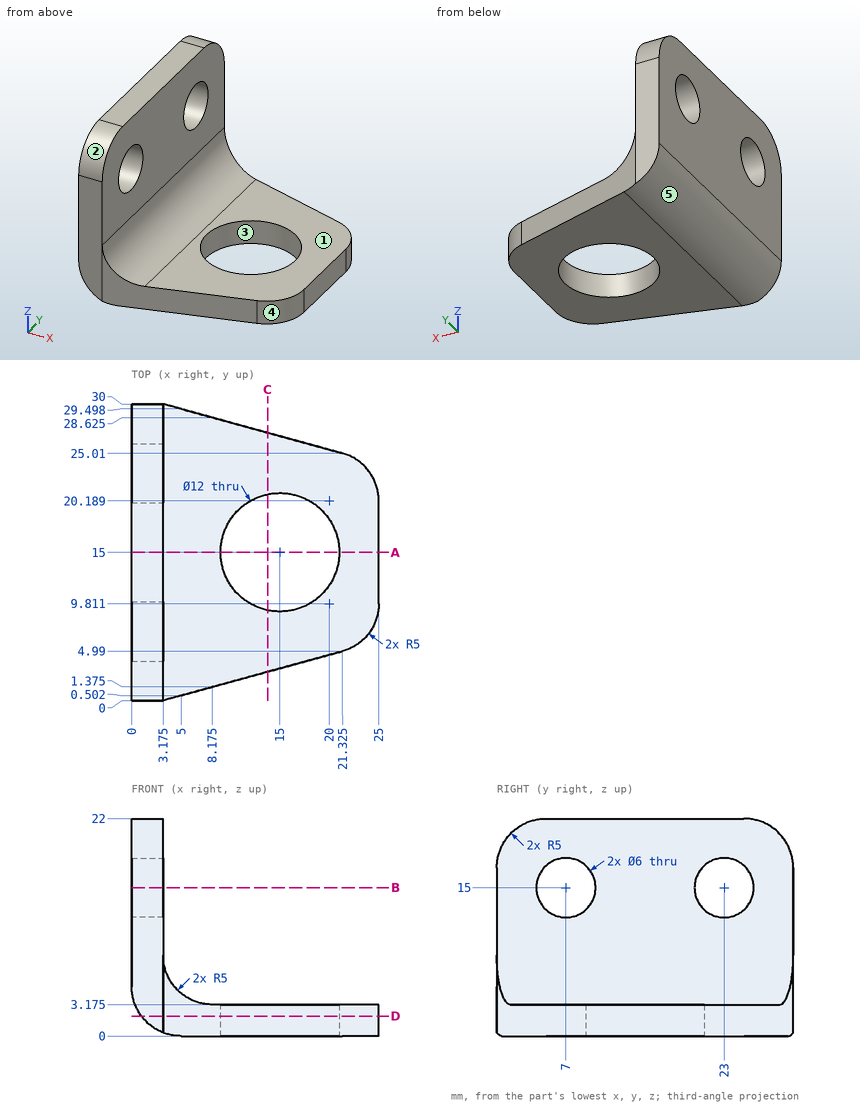
Verification items for this drawing (mm, ordinates from the low corner). A direction names the side the tool comes from. Coordinates: 2 decimals unless noted, no trailing zeros. Loops run counter-clockwise (first coordinate to the right, second up) from the corner with the lowest first, then second, coordinate; pieces in that order, holes last. Notation, with made-up numbers: (76, 10) - (123, 10) arc R5 ccw to (123, 18) - close; hole circle Ø9 at (73.5, 51). An arc over 180 degrees is marked (long way). Use one line per item in the form item = value. Start each with the question number.
Item 1: Gauge pin test, flat ends, axial feed: pin 1 (8 mm diameter, centred on x = 14.5, y = 18.5, fed in from +Z) (3 decimals); pin 2 (8 mm diameter, centred on y = 7, z = 15, fed in from +X) (3 decimals); pin 3 (12 mm diameter, centred on x = 15, z = 15.5, fed in from -Y); pin 4 (5 mm diameter, centred on y = 8, z = 6.5, fed in from +X) (1 decimal). Record the tip position at first contact, or that the pin passes through.
Item 2: Mould release check, pull along X, two halves, no side actions. Record for the marked faces 3, 4 and 5: +X half, -X half, draft (parallel to the pull), parting line (faces both ways), or undercut.
Item 3: Thickness scan on probe 1 along Y at (x, z) = (2.1, 15); probe 2 along X at (y, z) = (8, 19.5) (1 decimal). Record the ranges inside material, lowest first.
Item 4: Section check B-B, the plane z = 15. Enter the section's corners in (x, y) (1 decimal).
Item 5: Section check D-D, the plane z = 2. Enter the section's corners in (x, y) (1 decimal).
Item 6: Tool access check on the marked faces 1 and 2. Record the directions out of +Z, -Z, +X, -X, +Y, -Y that give a thin tool (end or side, any length) a straight path to the whole face; none if there is none.
Item 7: Section check C-C, the plane x = 13.75. Enter the section's corners in (y, z) (1 decimal).
Item 8: Section check A-A, the plane y = 15. Enter the section's corners in (x, z) (1 decimal), and give its area (3 significant figures).
Computed:
q1.pin_1 = 3.175
q1.pin_2 = 3.175
q1.pin_3 = through
q1.pin_4 = 5.4
q2.face_3 = undercut
q2.face_4 = +X half
q2.face_5 = -X half
q3.probe_1 = 0 to 4, 10 to 20, 26 to 30
q3.probe_2 = 0 to 3.2
q4.outline = (0, 0) - (3.2, 0) - (3.2, 4) - (0, 4) - close; (0, 10) - (3.2, 10) - (3.2, 20) - (0, 20) - close; (0, 26) - (3.2, 26) - (3.2, 30) - (0, 30) - close
q5.outline = (1, 0) - (3.2, 0) - (21.3, 5) arc R5 ccw to (25, 9.8) - (25, 20.2) arc R5 ccw to (21.3, 25) - (3.2, 30) - (1, 30) - close; hole circle Ø12 at (15, 15)
q6.face_1 = +Z, +X, +Y, -Y
q6.face_2 = +Z, +X, -X, -Y
q7.outline = (2.9, 0) - (9.1, 0) - (9.1, 3.2) - (2.9, 3.2) - close; (20.9, 0) - (27.1, 0) - (27.1, 3.2) - (20.9, 3.2) - close
q8.outline = (0, 5) arc R5 ccw to (5, 0) - (9, 0) - (9, 3.2) - (8.2, 3.2) arc R5 cw to (3.2, 8.2) - (3.2, 22) - (0, 22) - close; (21, 0) - (25, 0) - (25, 3.2) - (21, 3.2) - close
q8.area = 101 mm2
